from build123d import *

# Parameters (mm, degrees)
F0_R     = 4
F1_DEPTH = 5


with BuildPart() as f1:
    # F0 (on Top) → F1 (new body)
    with BuildSketch(Plane.XY):
        with BuildLine():
            Line((8, 24.799194), (8, 32))
            ThreePointArc((8, 32), (0, 40), (-8, 32))
            Line((-8, 32), (-8, 24.799194))
            ThreePointArc((-8, 24.799194), (-8.721733, 22.211448), (-10.678571, 20.370766))
            ThreePointArc((-10.678571, 20.370766), (-13.519061, 18.607391), (-16.07389, 16.450838))
            ThreePointArc((-16.07389, 16.450838), (-18.429178, 15.158575), (-21.113299, 15.271824))
            Line((-21.113299, 15.271824), (-27.961673, 17.496996))
            ThreePointArc((-27.961673, 17.496996), (-38.042261, 12.36068), (-32.905944, 2.280092))
            Line((-32.905944, 2.280092), (-26.057571, 0.05492))
            ThreePointArc((-26.057571, 0.05492), (-23.819506, -1.431146), (-22.67361, -3.861012))
            ThreePointArc((-22.67361, -3.861012), (-21.8743, -7.107391), (-20.612782, -10.203589))
            ThreePointArc((-20.612782, -10.203589), (-20.111591, -12.842933), (-21.048736, -15.360687))
            Line((-21.048736, -15.360687), (-25.281264, -21.186262))
            ThreePointArc((-25.281264, -21.186262), (-23.51141, -32.36068), (-12.336992, -30.590826))
            Line((-12.336992, -30.590826), (-8.104464, -24.765251))
            ThreePointArc((-8.104464, -24.765251), (-5.999531, -23.095944), (-3.33449, -22.757003))
            ThreePointArc((-3.33449, -22.757003), (0, -23), (3.33449, -22.757003))
            ThreePointArc((3.33449, -22.757003), (5.999531, -23.095944), (8.104464, -24.765251))
            Line((8.104464, -24.765251), (12.336992, -30.590826))
            ThreePointArc((12.336992, -30.590826), (23.51141, -32.36068), (25.281264, -21.186262))
            Line((25.281264, -21.186262), (21.048736, -15.360687))
            ThreePointArc((21.048736, -15.360687), (20.111591, -12.842933), (20.612782, -10.203589))
            ThreePointArc((20.612782, -10.203589), (21.8743, -7.107391), (22.67361, -3.861012))
            ThreePointArc((22.67361, -3.861012), (23.819506, -1.431146), (26.057571, 0.05492))
            Line((26.057571, 0.05492), (32.905944, 2.280092))
            ThreePointArc((32.905944, 2.280092), (38.042261, 12.36068), (27.961673, 17.496996))
            Line((27.961673, 17.496996), (21.113299, 15.271824))
            ThreePointArc((21.113299, 15.271824), (18.429178, 15.158575), (16.07389, 16.450838))
            ThreePointArc((16.07389, 16.450838), (13.519061, 18.607391), (10.678571, 20.370766))
            ThreePointArc((10.678571, 20.370766), (8.721733, 22.211448), (8, 24.799194))
        make_face()
        with Locations((-18.809128, -25.888544)):
            Circle(F0_R, mode=Mode.SUBTRACT)
        with Locations((18.809128, -25.888544)):
            Circle(F0_R, mode=Mode.SUBTRACT)
        Polygon((0, -15.011107), (-13, -7.505553), (-13, 7.505553), (0, 15.011107), (13, 7.505553), (13, -7.505553), align=None, mode=Mode.SUBTRACT)
        with Locations((-30.433809, 9.888544)):
            Circle(F0_R, mode=Mode.SUBTRACT)
        with Locations((30.433809, 9.888544)):
            Circle(F0_R, mode=Mode.SUBTRACT)
        with Locations((0, 32)):
            Circle(F0_R, mode=Mode.SUBTRACT)
    extrude(amount=F1_DEPTH)


solid = f1.part
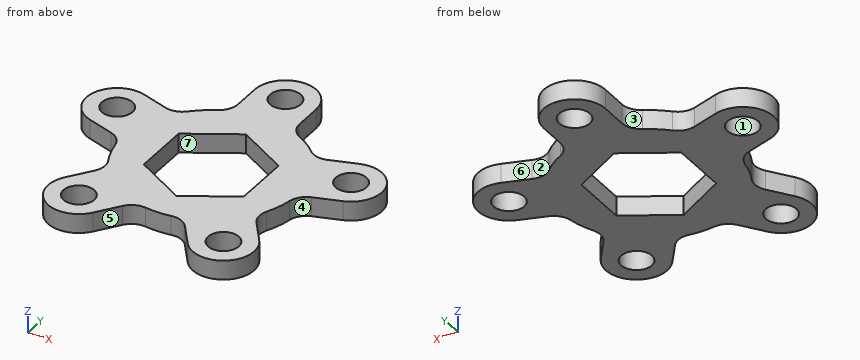
Check sheet for the modelled part. Datum: model origin and axes. Units: mm. Face numbers are marked on the shaded views. A direction names the side the tool comes from. Round coordinates to 2 decimals unless told otherwise and drop trailing zeros. Loops run counter-clockwise (first coordinate to the right, second up) from the corner with the lowest first, then second, coordinate; pieces in that order, holes last.
1. Set-up check for the marked faces 5, 6 and 7: record each of +Z, -Z, +X, -X, +Y, -Y from which the full face is reachable in a straight line by a thin tool's end or side.
2. Sectioned sample at A-A on y = -1.5. Record the boundary of the cut face in (x, z), and give its area (3 significant figures).
3. Gauge pin test, flat ends, axial feed: pin 1 Ø5 at (x, y) = (-30.43, 9.89) entering from +Z; pin 2 Ø2.5 at (y, z) = (28.5, 1.5) entering from -X; pin 3 Ø2.5 at (y, z) = (28.5, 1.5) entering from +X; pin 4 Ø1.5 at (y, z) = (8.5, 3.5) entering from -X. Record the tip position at first contact, or that the pin passes through.
4. Sectioned sample at C-C on y = 19. Record the boundary of the cut face in (x, z), and give its area (3 significant figures).
5. Mould release check, pull along X, two halves, no side actions. Record for the marked faces 1, 2, 3 and 4: released by +X, released by -X, zero draft, split by the parting line, or undercut.
6. Sectioned sample at D-D on y = -16.5. Record the boundary of the cut face in (x, z).
7. Scan lines: probe 1 along Y at (x, z) = (-0.5, 4.3); probe 2 along X at (y, z) = (9.5, 4.2); probe 3 along X at (y, z) = (-26.5, 4.7). Record each from-to range of solid material in increasing order.
8. Sectioned sample at B-B on z = 1.3. Give the number of separate pieces and of enclosed holes in the cut face, and give its area (3 significant figures).
Recorded:
1. face 5: +Z, -Z, -Y
1. face 6: +Z, -Z, +Y
1. face 7: +Z, -Z
2. outline: (-23.76, 0) - (-13, 0) - (-13, 5) - (-23.76, 5) - close; (13, 0) - (23.76, 0) - (23.76, 5) - (13, 5) - close
2. area: 108 mm2
3. pin 1: passes through
3. pin 2: stops at x = -8
3. pin 3: stops at x = 8
3. pin 4: stops at x = -38.41
4. outline: (-12.96, 0) - (12.96, 0) - (12.96, 5) - (-12.96, 5) - close
4. area: 130 mm2
5. face 1: undercut
5. face 2: undercut
5. face 3: released by -X
5. face 4: released by +X
6. outline: (-21.88, 0) - (21.88, 0) - (21.88, 5) - (-21.88, 5) - close
7. probe 1: y = -22.99 to -14.72, 14.72 to 28.03, 35.97 to 39.98
7. probe 2: x = -38.42 to -34.41, -26.45 to -9.55, 9.55 to 26.45, 34.41 to 38.42
7. probe 3: x = -26.79 to -22.76, -14.86 to -9.36, 9.36 to 14.86, 22.76 to 26.79
8. separate pieces: 1
8. enclosed holes: 6
8. area: 2,100 mm2
